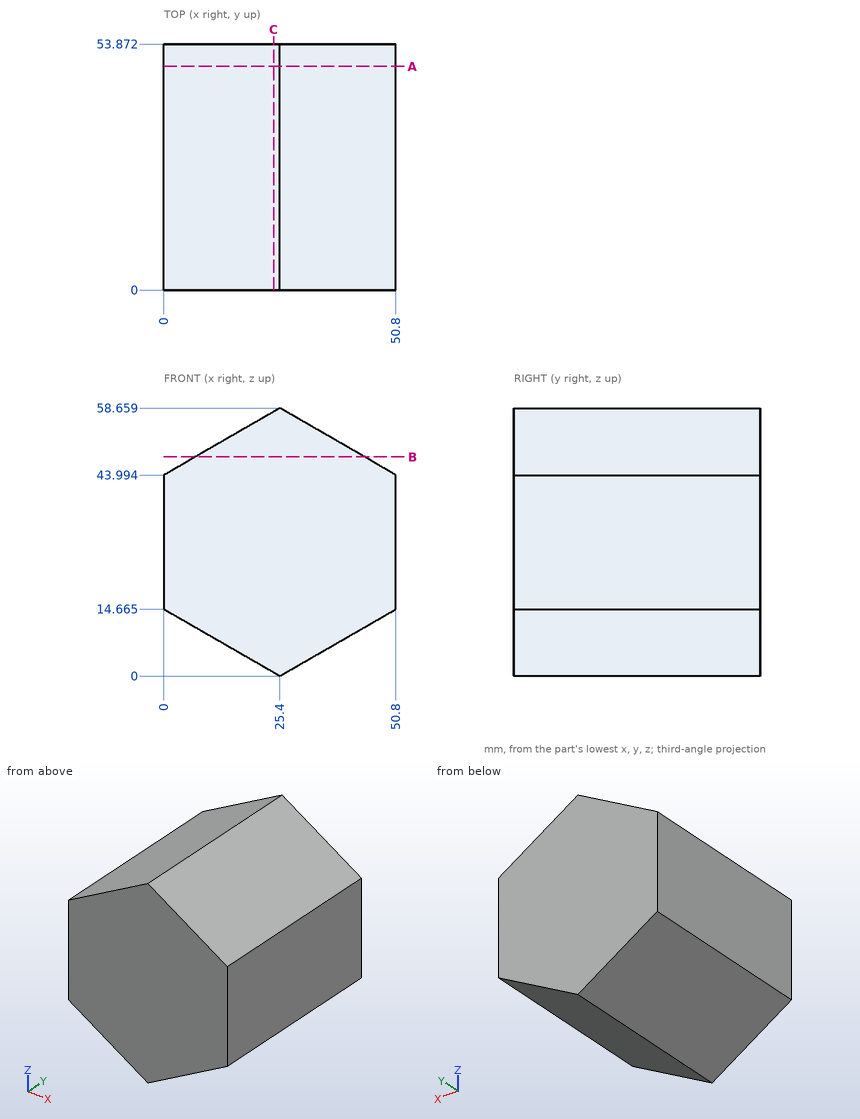
The drawing under review shows one solid part. Ordinate dimensions are in mm from its lowest x, y, z. Coordinates: 2 decimals unless noted, no trailing zeros. Loops run counter-clockwise (first coordinate to the right, second up) from the corner with the lowest first, then second, coordinate; pieces in that order, holes last.
Item 1: Add section A-A (y = 49). Write out the cut boundary in (x, z) (1 decimal).
Completed:
outline: (0, 14.7) - (25.4, 0) - (50.8, 14.7) - (50.8, 44) - (25.4, 58.7) - (0, 44) - close
Item 2: Add section C-C (x = 24). Write out the cut boundary in (y, z).
Completed:
outline: (0, 0.81) - (53.87, 0.81) - (53.87, 57.85) - (0, 57.85) - close
Item 3: Wall thickness on L1, parallel to X at y = 44.5, z = 47 (1 decimal); L2, parallel to Z at x = 35, y = 27 (1 decimal); L3, parallel to Z at x = 48.5, y = 24.5: over which ranges is each line inside the solid? List them lowest first.
Completed:
L1: x = 5.2 to 45.6
L2: z = 5.5 to 53.1
L3: z = 13.34 to 45.32
Item 4: Add section B-B (z = 48). Write out the cut boundary in (x, y), and give its area (3 significant figures).
Completed:
outline: (6.94, 0) - (43.86, 0) - (43.86, 53.87) - (6.94, 53.87) - close
area: 1,990 mm2
Item 5: Clearance check with flat-ended pins moving along their axes: pin 1 (1 mm diameter, centred on y = 26, z = 46.5, fed in from +X) (1 decimal); pin 2 (10 mm diameter, centred on x = 43, y = 20, fed in from +Z) (1 decimal); pin 3 (10 mm diameter, centred on x = 31.5, y = 26, fed in from +Z). State where each tip first meets the part, or that it passes through.
Completed:
pin 1: stops at x = 47.3
pin 2: stops at z = 51.4
pin 3: stops at z = 58.02
